Verification items for the finished model (mm, model axes). Face numbers are marked on the shaded views. A direction names the side the tool comes from. Give positions to 0.01 mm unless a question says otherwise; leave off trailing zeros. Write each loop counter-clockwise with the first axis right and the second up, starting at its lowest first coordinate (ties: lowest second). Pieces come first, ordered by that corner, then holes. Notation, with made-up numbers: M 12,60 L 28,60 A20 ccw 28,96 Z; hole C -7,20.25 d3. An arc over 180 degrees is marked long. Write item = value, one per line.
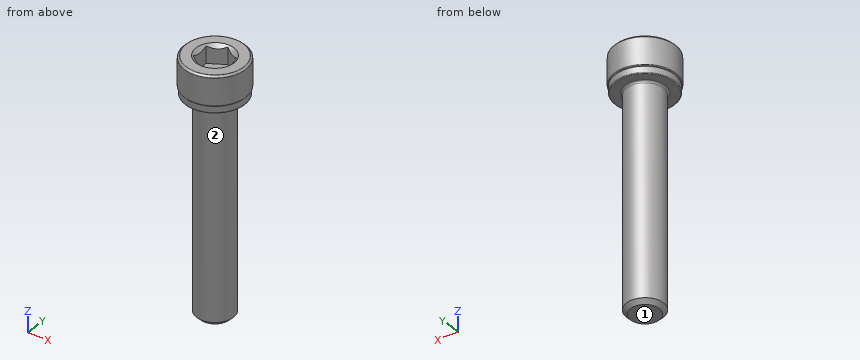
from build123d import *

# Parameters (mm, degrees)
CUT_EXTRUDE1_START = -3
CUT_EXTRUDE1_DEPTH = 3
SKETCH4_R          = 3.103257697
CUT_EXTRUDE2_DEPTH = 3
CUT_EXTRUDE2_TAPER = 45


with BuildPart() as part:
    # Sketch2 → Revolve1 (revolve)
    with BuildSketch(Plane(origin=(0, 0, 0), x_dir=(0, 0, -1), z_dir=(1, 0, 0))):
        with BuildLine():
            Line((-20.5, 0), (-20.5, 4.661167479))
            ThreePointArc((-20.5, 4.661167479), (-20.492863706, 4.69704405), (-20.472541261, 4.727458739))
            Line((-20.472541261, 4.727458739), (-20.227458739, 4.972541261))
            ThreePointArc((-20.227458739, 4.972541261), (-20.19704405, 4.992863706), (-20.161167479, 5))
            Line((-20.161167479, 5), (-15.813832521, 5))
            ThreePointArc((-15.813832521, 5), (-15.77795595, 4.992863706), (-15.747541261, 4.972541261))
            Line((-15.747541261, 4.972541261), (-15.652458739, 4.877458739))
            ThreePointArc((-15.652458739, 4.877458739), (-15.62204405, 4.857136294), (-15.586167479, 4.85))
            Line((-15.586167479, 4.85), (-14.625, 4.85))
            ThreePointArc((-14.625, 4.85), (-14.536611652, 4.813388348), (-14.5, 4.725))
            Line((-14.5, 4.725), (-14.5, 3.3))
            ThreePointArc((-14.5, 3.3), (-14.412132034, 3.087867966), (-14.2, 3))
            Line((-14.2, 3), (19.850480947, 3))
            Line((19.850480947, 3), (20.5, 2.350480947))
            Line((20.5, 2.350480947), (20.5, 0))
            Line((20.5, 0), (-20.5, 0))
        make_face()
    revolve(axis=Axis((0, 0, -20.5), (0, 0, 1)))

    # Sketch3 → Cut-Extrude1 (cut)
    with BuildSketch(Plane.XY.offset(20.5).offset(CUT_EXTRUDE1_START)):
        Polygon((2.5, -1.443375673), (2.5, 1.443375673), (0, 2.886751346), (-2.5, 1.443375673), (-2.5, -1.443375673), (0, -2.886751346), align=None)
    extrude(amount=CUT_EXTRUDE1_DEPTH, mode=Mode.SUBTRACT)

    # Sketch4 → Cut-Extrude2 (cut)
    with BuildSketch(Plane.XY.offset(20.5)):
        Circle(SKETCH4_R)
    extrude(amount=-CUT_EXTRUDE2_DEPTH, taper=CUT_EXTRUDE2_TAPER, mode=Mode.SUBTRACT)


solid = part.part
1) Cross-section at A-A on z = 17. Record the boundary of the cut face in (x, y).
From the geometry:
outline = C 0,0 d10
2) Tool access check on the marked faces 1 and 2. Record the directions out of +Z, -Z, +X, -X, +Y, -Y that give a thin tool (end or side, any length) a straight path to the whole face; none if there is none.
From the geometry:
face_1 = -Z, +X, -X, +Y, -Y
face_2 = -Z
3) Cross-section at B-B on z = 3. Record the boundary of the cut face in (x, y), plus the area to 3 significant figures.
From the geometry:
outline = C 0,0 d6
area = 28.3 mm^2
4) Depth check by flat-ended pin: P1, Ø2.5, axis at x = 0.5, y = 0, coming from the +Z side; P2, Ø1, axis at x = -2, z = -12, coming from the +Y side; P3, Ø1.5, axis at y = -1, z = -15, coming from the +X side. Enter the tip coordinate at first touch or a pass-through.
From the geometry:
P1 = 17.5
P2 = 2.6
P3 = 2.99
5) Material ranges on probe 1 along Z at (x, y) = (2.5, 3.75); probe 2 along Z at (x, y) = (2, 1); probe 3 along Y at (x, z) = (1, 18.5), recorded low to high. Write a range as from..to.
From the geometry:
probe_1 = 14.5..20.5
probe_2 = -20.5..17.5
probe_3 = -4.9..-2.31, 2.31..4.9
